from build123d import *

# Parameters (mm, degrees)
BOSS_EXTRUDE1_DEPTH = 17.5
FILLET3_R           = 10
SKETCH2_R           = 22.5
BOSS_EXTRUDE4_DEPTH = 10
SKETCH4_R           = 3
CUT_EXTRUDE2_DEPTH  = 10
FILLET6_R           = 15
SKETCH6_R           = 4.5
CUT_EXTRUDE3_DEPTH  = 84.517962215


with BuildPart() as part:
    # Sketch1 → Boss-Extrude1 (new, symmetric)
    with BuildSketch(Plane.XY):
        Polygon((-31.5, 0), (31.5, 0), (31.5, 50), (27, 50), (27, 10), (-27, 10), (-27, 50), (-31.5, 50), align=None)
    extrude(amount=BOSS_EXTRUDE1_DEPTH, both=True)

    # Fillet3
    fillet3_edges = [part.edges().sort_by_distance(p)[0] for p in [
        (-27, 10, 0),
        (27, 10, 0),
        (31.5, 0, 0),
        (-31.5, 0, 0),
    ]]
    fillet(fillet3_edges, radius=FILLET3_R)

    # Sketch2 → Boss-Extrude4 (add)
    with BuildSketch(Plane.XZ):
        Circle(SKETCH2_R)
    extrude(amount=-BOSS_EXTRUDE4_DEPTH)

    # Sketch4 → Cut-Extrude2 (cut)
    with BuildSketch(Plane.XZ):
        with Locations((0, 13)):
            Circle(SKETCH4_R)
        with Locations((13, 0)):
            Circle(SKETCH4_R)
        with Locations((0, -13)):
            Circle(SKETCH4_R)
        with Locations((-13, 0)):
            Circle(SKETCH4_R)
    extrude(amount=-CUT_EXTRUDE2_DEPTH, mode=Mode.SUBTRACT)

    # Fillet6
    fillet6_edges = [part.edges().sort_by_distance(p)[0] for p in [
        (29.25, 50, 17.5),
        (29.25, 50, -17.5),
        (-29.25, 50, -17.5),
        (-29.25, 50, 17.5),
    ]]
    fillet(fillet6_edges, radius=FILLET6_R)

    # Sketch6 → Cut-Extrude3 (cut, through all)
    with BuildSketch(Plane(origin=(31.5, 0, 0), x_dir=(0, 0, -1), z_dir=(1, 0, 0))):
        with Locations(Location((0, 39, 0), (0, 0, 90))):
            Circle(SKETCH6_R)
    extrude(amount=-CUT_EXTRUDE3_DEPTH, mode=Mode.SUBTRACT)


solid = part.part
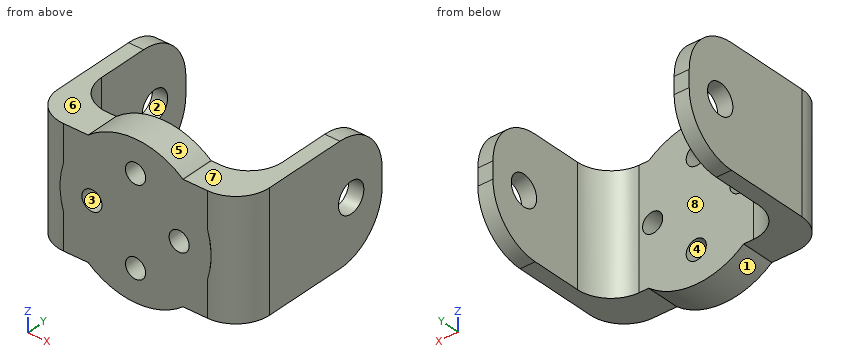
Can you work these out from the model? Positions are in its coordinate system, mm. Face numbers are marked on the shaded views. A direction names the side the tool comes from. Round coordinates to 2 decimals unless told otherwise and drop trailing zeros. Order: outer loops, then holes, each group sorted by start corner. A loop starts at its lowest first (then second) coordinate and runs counter-clockwise, first axis right, second up. Notation, with made-up numbers: M -35.75,-21 L -15.75,-21 A9 ccw -15.75,-7 Z; hole C -32.75,23.5 d3. An arc over 180 degrees is marked long. Use a Markdown table: item, result.
1) If I drill on line 1 along Z through (x, y) = (0, 6); line 2 along X through (y, z) = (40.5, 7.5); line 3 along Y through (x, z) = (-17, 12), over which ranges is the centre line in solid material (lowest first)?
Geometry says:
| item | result |
|---|---|
| line 1 | z = -22.5 to -16, -10 to 10, 16 to 22.5 |
| line 2 | x = -31.5 to -27, 27 to 31.5 |
| line 3 | y = 0 to 10 |
2) I'm going to push flat-ended pins straight in: P1, Ø17, axis at x = 5, z = -10.5, coming from the +Y side; P2, Ø1.5, axis at x = -23, z = 6.5, coming from the +Y side; P3, Ø1, axis at x = -7.5, z = -17.5, coming from the -Y side; P4, Ø19, axis at x = 19.5, y = 21, coming from the +Z side. Where does each tip first touch, or does it pass through?
Geometry says:
| item | result |
|---|---|
| P1 | stops at y = 10 |
| P2 | stops at y = 12.62 |
| P3 | stops at y = 0 |
| P4 | stops at z = 17.5 |
3) Imagine slicing it at D-D (x = -13). List the corners of the cut face in (y, z) for me, then the cut area to 3 significant figures.
Geometry says:
| item | result |
|---|---|
| outline | M 0,-18.36 L 10,-18.36 L 10,-3 L 0,-3 Z; M 0,3 L 10,3 L 10,18.36 L 0,18.36 Z |
| area | 307 mm² |
4) If we mould it in two halves opening along X, with no side actions, what happens to the marked faces 1, 2, 3 and 4? For each: +X half, -X half, draft (parallel to the pull), parting line (faces both ways), or undercut.
Geometry says:
| item | result |
|---|---|
| face 1 | parting line |
| face 2 | draft |
| face 3 | undercut |
| face 4 | undercut |
5) On a 3-axis mill with a long thin cutter (end or side, diameter ignored), from which of +Z, -Z, +X, -X, +Y, -Y can I reach the whole of each face in a straight line? I mean the marked faces 5, 6, 7 and 8. Say none if no direction works.
Geometry says:
| item | result |
|---|---|
| face 5 | +Z, +Y, -Y |
| face 6 | +Z, -X, +Y, -Y |
| face 7 | +Z, +X, +Y, -Y |
| face 8 | +Z, -Z, +Y |
6) Imagine slicing it at C-C (z = 13). List the corners of the cut face in (x, y) for me.
Geometry says:
| item | result |
|---|---|
| outline | M -31.5,10 A10 ccw -21.5,0 L -3,0 L -3,10 L -17,10 A10 cw -27,20 L -27,45.71 L -31.5,45.71 Z; M 3,0 L 21.5,0 A10 ccw 31.5,10 L 31.5,45.71 L 27,45.71 L 27,20 A10 cw 17,10 L 3,10 Z |
7) Imagine slicing it at B-B (x = 0). List the corners of the cut face in (y, z) for me.
Geometry says:
| item | result |
|---|---|
| outline | M 0,-22.5 L 10,-22.5 L 10,-16 L 0,-16 Z; M 0,-10 L 10,-10 L 10,10 L 0,10 Z; M 0,16 L 10,16 L 10,22.5 L 0,22.5 Z |
8) Imagine slicing it at A-A (y = 27). List the corners of the cut face in (x, z) for me, then the cut area to 3 significant figures.
Geometry says:
| item | result |
|---|---|
| outline | M -31.5,-17.5 L -27,-17.5 L -27,17.5 L -31.5,17.5 Z; M 27,-17.5 L 31.5,-17.5 L 31.5,17.5 L 27,17.5 Z |
| area | 315 mm² |
